from build123d import *

# Parameters (mm, degrees)
BOSS_EXTRUDE1_DEPTH   = 3.175
F_6_CLEARANCE_HOLE1_D = 4.3053
F_2_CLEARANCE_HOLE1_D = 2.7051
FILLET1_R             = 3.175
FILLET2_R             = 6.35


with BuildPart() as part:
    # Sketch1 → Boss-Extrude1 (new body)
    with BuildSketch(Plane.XY):
        with BuildLine():
            Line((0, 3.175), (-40.698258, 3.175))
            Line((-40.698258, 3.175), (-40.698258, -50.175))
            Line((-40.698258, -50.175), (0, -50.175))
            ThreePointArc((0, -50.175), (2.24506403, -49.24506403), (3.175, -47))
            Line((3.175, -47), (3.175, 0))
            ThreePointArc((3.175, 0), (2.24506403, 2.24506403), (0, 3.175))
        make_face()
        with BuildLine():
            Line((-34.348258, -3.175), (-23, -3.175))
            ThreePointArc((-23, -3.175), (-20.75493597, -2.24506403), (-19.825, 0))
            Line((-19.825, 0), (-3.175, 0))
            Line((-3.175, 0), (-3.175, -47))
            Line((-3.175, -47), (-19.825, -47))
            ThreePointArc((-19.825, -47), (-20.75493597, -44.75493597), (-23, -43.825))
            Line((-23, -43.825), (-34.348258, -43.825))
            Line((-34.348258, -43.825), (-34.348258, -3.175))
        make_face(mode=Mode.SUBTRACT)
    extrude(amount=BOSS_EXTRUDE1_DEPTH)

    # #6 Clearance Hole1 (through all)
    with Locations(Plane.XY.offset(3.175)):
        with Locations((-37.523258, -26.062402)):
            Hole(F_6_CLEARANCE_HOLE1_D / 2)

    # #2 Clearance Hole1 (through all)
    with Locations(Plane.XY.offset(3.175)):
        with Locations((-23, -47), (0, -47), (0, 0), (-23, 0), (0, -24)):
            Hole(F_2_CLEARANCE_HOLE1_D / 2)

    # Fillet1
    fillet1_edges = [part.edges().sort_by_distance(p)[0] for p in [
        (-3.175, -47, 1.5875),
        (-3.175, 0, 1.5875),
        (-19.825, 0, 1.5875),
        (-19.825, -47, 1.5875),
    ]]
    fillet(fillet1_edges, radius=FILLET1_R)

    # Fillet2
    fillet2_edges = [part.edges().sort_by_distance(p)[0] for p in [
        (-40.698258, -50.175, 1.5875),
        (-40.698258, 3.175, 1.5875),
        (-34.348258, -3.175, 1.5875),
        (-34.348258, -43.825, 1.5875),
    ]]
    fillet(fillet2_edges, radius=FILLET2_R)


solid = part.part
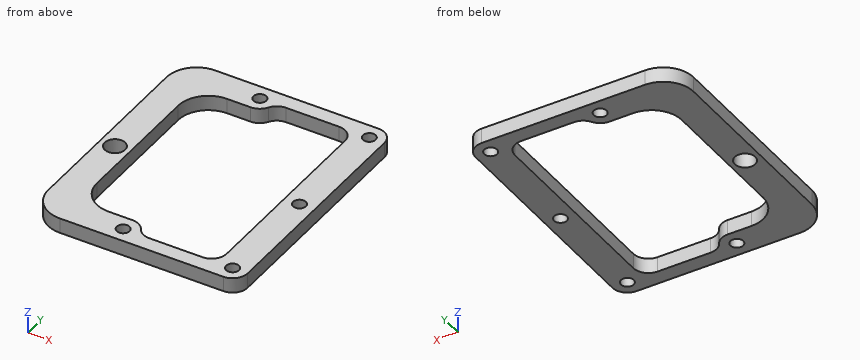
Source: CAD feature listing. Evaluate the final solid. Frame: model axes, mm. Round coordinates to 2 decimals unless told otherwise and drop trailing zeros. Loops run counter-clockwise (first coordinate to the right, second up) from the corner with the lowest first, then second, coordinate; pieces in that order, holes last.
Q1. Section C-C, the plane z = 0.6. State how many separate pieces and enclosed holes the cut face has, plus the area to 3 significant figures.
Q2. Ray query, line 1 (Y direction, x = -23, z = 1.45) (3 decimals); line 2 (X direction, y = -26, z = 2.05) (3 decimals); line 3 (Y direction, x = -16.5, z = 1.85) (3 decimals). Return the intervals inside material, ascending.
Q3. Section A-A, the plane y = -6. Return loops of the section in (x, z) (3 decimals).
Q4. Section B-B, the plane x = -25. Return loops of the section in (y, z) (3 decimals).
Solutions:
1. separate pieces: 1
1. enclosed holes: 7
1. area: 922 mm2
2. line 1: y = -50.175 to -48.353, -45.647 to -43.825, -3.175 to -1.353, 1.353 to 3.175
2. line 2: x = -40.698 to -39.675, -35.372 to -34.348, -3.175 to 3.175
2. line 3: y = -50.175 to -47, 0 to 3.175
3. outline: (-40.698, 0) - (-33.28, 0) - (-33.28, 3.175) - (-40.698, 3.175) - close; (-3.175, 0) - (3.175, 0) - (3.175, 3.175) - (-3.175, 3.175) - close
4. outline: (-50.175, 0) - (-43.825, 0) - (-43.825, 3.175) - (-50.175, 3.175) - close; (-3.175, 0) - (3.175, 0) - (3.175, 3.175) - (-3.175, 3.175) - close
